The listing builds one solid part. Answer for the finished solid, in the listing's coordinates (mm). Coordinates: 2 decimals unless noted, no trailing zeros. Loops run counter-clockwise (first coordinate to the right, second up) from the corner with the lowest first, then second, coordinate; pieces in that order, holes last. Notation, with made-up numbers: (13, 22) - (36, 22) arc R20 cw to (36, 56) - close; hole circle Ø10 at (49.5, 62.5). An arc over 180 degrees is marked (long way). Put each result on its own line as item: value.
```python
from build123d import *

# Parameters (mm, degrees)
BOSS_EXTRUDE1_DEPTH = 0.25
SKETCH4_R           = 0.25
CUT_EXTRUDE1_DEPTH  = 9.5


with BuildPart() as part:
    # Sketch2 → Boss-Extrude1 (new, symmetric)
    with BuildSketch(Plane.XY):
        with BuildLine():
            Line((-7.074484682, 38.444256199), (-7.074484682, 37.916334323))
            Line((-7.074484682, 37.916334323), (-7.200133049, 37.916334323))
            ThreePointArc((-7.200133049, 37.916334323), (-7.828750978, 37.655952251), (-8.089133049, 37.027334323))
            Line((-8.089133049, 37.027334323), (-8.089133049, 26.105334323))
            ThreePointArc((-8.089133049, 26.105334323), (-7.828750978, 25.476716394), (-7.200133049, 25.216334323))
            Line((-7.200133049, 25.216334323), (-6.313836315, 25.216334323))
            ThreePointArc((-6.313836315, 25.216334323), (-5.685218387, 25.476716394), (-5.424836315, 26.105334323))
            Line((-5.424836315, 26.105334323), (-5.424836315, 37.027334323))
            ThreePointArc((-5.424836315, 37.027334323), (-5.685218387, 37.655952251), (-6.313836315, 37.916334323))
            Line((-6.313836315, 37.916334323), (-6.439484682, 37.916334323))
            Line((-6.439484682, 37.916334323), (-6.439484682, 38.444256199))
            ThreePointArc((-6.439484682, 38.444256199), (-6.756984682, 43.504334323), (-7.074484682, 38.444256199))
        make_face()
    extrude(amount=BOSS_EXTRUDE1_DEPTH, both=True)

    # Sketch4 → Cut-Extrude1 (cut)
    with BuildSketch(Plane.XY.offset(0.25)):
        with Locations((-7.514442014, 25.791025359)):
            Circle(SKETCH4_R)
        with Locations((-5.999527351, 25.791025359)):
            Circle(SKETCH4_R)
        with Locations((-7.514442014, 37.341643287)):
            Circle(SKETCH4_R)
        with Locations((-5.999527351, 37.341643287)):
            Circle(SKETCH4_R)
    extrude(amount=-CUT_EXTRUDE1_DEPTH, mode=Mode.SUBTRACT)


solid = part.part
```
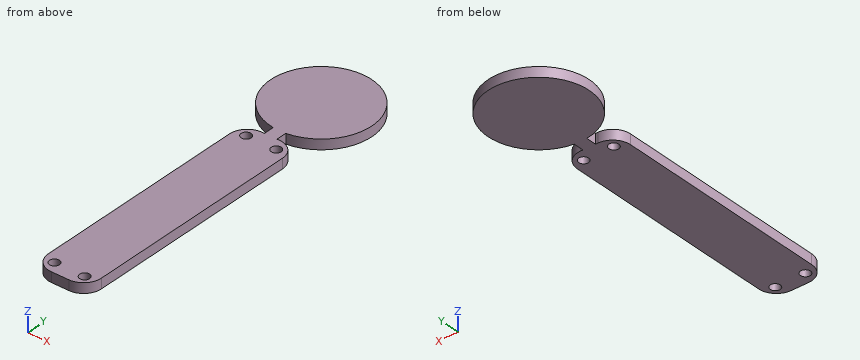
1) Straight lines are drawn through the part: L1, parallel to X at y = 37.25, z = 0; L2, parallel to Y at x = -6.05, z = -0.2; L3, parallel to X at y = 37.5, z = -0.1. For each, find the intervals that lie inside material, in ascending order. Write a range as [from, to].
Found:
L1: x = [-8.06, -7.75], [-7.28, -6.23], [-5.77, -5.45]
L2: y = [25.26, 25.55], [26.04, 37.1], [37.59, 37.88], [38.52, 43.4]
L3: x = [-7.95, -7.71], [-7.32, -6.19], [-5.81, -5.56]
2) The part is cut by section A-A (x = -7.6). Give the vertices of the cut face in (y, z), and give its area (3 significant figures).
Found:
outline: (25.31, -0.25) - (25.56, -0.25) - (25.56, 0.25) - (25.31, 0.25) - close; (26.03, -0.25) - (37.11, -0.25) - (37.11, 0.25) - (26.03, 0.25) - close; (37.58, -0.25) - (37.82, -0.25) - (37.82, 0.25) - (37.58, 0.25) - close; (38.57, -0.25) - (43.36, -0.25) - (43.36, 0.25) - (38.57, 0.25) - close
area: 8.18 mm^2
3) The part is cut by section D-D (x = -4.75). Give the vertices of the cut face in (y, z), and give its area (3 significant figures).
Found:
outline: (39.41, -0.25) - (42.52, -0.25) - (42.52, 0.25) - (39.41, 0.25) - close
area: 1.56 mm^2
4) The part is cut by section C-C (y = 35.25). Give the vertices of the cut face in (x, z).
Found:
outline: (-8.09, -0.25) - (-5.42, -0.25) - (-5.42, 0.25) - (-8.09, 0.25) - close
5) The part is cut by section B-B (z = 0). Give the vertices of the cut face in (x, y), and give its area (3 significant figures).
Found:
outline: (-8.09, 26.11) arc R0.89 ccw to (-7.2, 25.22) - (-6.31, 25.22) arc R0.89 ccw to (-5.42, 26.11) - (-5.42, 37.03) arc R0.89 ccw to (-6.31, 37.92) - (-6.44, 37.92) - (-6.44, 38.44) arc R2.54 ccw (long way) to (-7.07, 38.44) - (-7.07, 37.92) - (-7.2, 37.92) arc R0.89 ccw to (-8.09, 37.03) - close; hole circle Ø0.5 at (-7.51, 25.79); hole circle Ø0.5 at (-7.51, 37.34); hole circle Ø0.5 at (-6, 25.79); hole circle Ø0.5 at (-6, 37.34)
area: 53.0 mm^2
